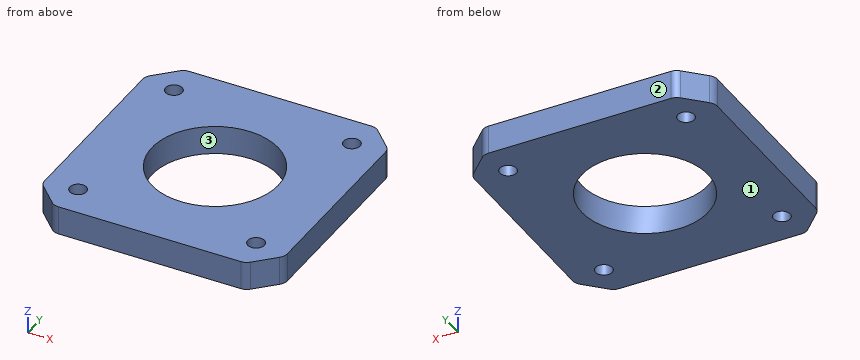
from build123d import *

# Parameters (mm, degrees)
SKETCH1_R           = 1.45
SKETCH1_R_2         = 11
BOSS_EXTRUDE1_DEPTH = 5


with BuildPart() as part:
    # Sketch1 → Boss-Extrude1 (new body)
    with BuildSketch(Plane.XY):
        with BuildLine():
            Line((-20.564213562, -17.28137085), (-17.28137085, -20.564213562))
            ThreePointArc((-17.28137085, -20.564213562), (-16.632524152, -20.997759065), (-15.867157288, -21.15))
            Line((-15.867157288, -21.15), (15.867157288, -21.15))
            ThreePointArc((15.867157288, -21.15), (16.632524152, -20.997759065), (17.28137085, -20.564213562))
            Line((17.28137085, -20.564213562), (20.564213562, -17.28137085))
            ThreePointArc((20.564213562, -17.28137085), (20.997759065, -16.632524152), (21.15, -15.867157288))
            Line((21.15, -15.867157288), (21.15, 15.867157288))
            ThreePointArc((21.15, 15.867157288), (20.997759065, 16.632524152), (20.564213562, 17.28137085))
            Line((20.564213562, 17.28137085), (17.28137085, 20.564213562))
            ThreePointArc((17.28137085, 20.564213562), (16.632524152, 20.997759065), (15.867157288, 21.15))
            Line((15.867157288, 21.15), (-15.867157288, 21.15))
            ThreePointArc((-15.867157288, 21.15), (-16.632524152, 20.997759065), (-17.28137085, 20.564213562))
            Line((-17.28137085, 20.564213562), (-20.564213562, 17.28137085))
            ThreePointArc((-20.564213562, 17.28137085), (-20.997759065, 16.632524152), (-21.15, 15.867157288))
            Line((-21.15, 15.867157288), (-21.15, -15.867157288))
            ThreePointArc((-21.15, -15.867157288), (-20.997759065, -16.632524152), (-20.564213562, -17.28137085))
        make_face()
        with Locations((-15.5, 15.5)):
            Circle(SKETCH1_R, mode=Mode.SUBTRACT)
        with Locations((15.5, 15.5)):
            Circle(SKETCH1_R, mode=Mode.SUBTRACT)
        with Locations((15.5, -15.5)):
            Circle(SKETCH1_R, mode=Mode.SUBTRACT)
        with Locations((-15.5, -15.5)):
            Circle(SKETCH1_R, mode=Mode.SUBTRACT)
        Circle(SKETCH1_R_2, mode=Mode.SUBTRACT)
    extrude(amount=BOSS_EXTRUDE1_DEPTH)


solid = part.part
Design review of the part built by this model. Coordinates are the model's own, in mm. Face numbers are marked on the shaded views. Give positions to 0.01 mm unless a question says otherwise; leave off trailing zeros. Write each loop counter-clockwise with the first axis right and the second up, starting at its lowest first coordinate (ties: lowest second). Pieces come first, ordered by that corner, then holes. Notation, with made-up numbers: M 87,29 L 129,29 A19 ccw 129,33 Z; hole C 21,36 d2. An arc over 180 degrees is marked long. Answer as a JSON object with one key per item and string values. Group by question number.
1) We need section A-A (y = 0). Give the boundary of the cut face in (x, z).
2) Mouldability with a two-part tool opening along Y and no side actions: class the marked faces 1, 2 and 3 as released by +Y, released by -Y, zero draft, split by the parting line, or undercut.
3) Clearance check with flat-ended pins moving along their axes: pin 1 Ø1 at (x, z) = (16, 4.5) entering from -Y; pin 2 Ø2.5 at (x, y) = (-15.5, -15.5) entering from -Z. State where each tip first meets the part, or that it passes through.
4) For line 1 along Y through (x, z) = (-15.5, 2.95); line 2 along Y through (x, z) = (0, 2); line 3 along Y through (x, z) = (-2.5, 2.6), list the stretches that pass through material, from the lowest coordinate up.
5) We need section C-C (z = 2.25). Give the boundary of the cut face in (x, y), and give its area (3 significant figures).
Answer key:
{
 "1": {"outline": "M -21.15,0 L -11,0 L -11,5 L -21.15,5 Z; M 11,0 L 21.15,0 L 21.15,5 L 11,5 Z"},
 "2": {"face 1": "zero draft", "face 2": "released by +Y", "face 3": "undercut"},
 "3": {"pin 1": "stops at y = -21.15", "pin 2": "passes through"},
 "4": {"line 1": "y = -21.15 to -16.95, -14.05 to 14.05, 16.95 to 21.15", "line 2": "y = -21.15 to -11, 11 to 21.15", "line 3": "y = -21.15 to -10.71, 10.71 to 21.15"},
 "5": {"outline": "M -21.15,-15.87 A2 ccw -20.56,-17.28 L -17.28,-20.56 A2 ccw -15.87,-21.15 L 15.87,-21.15 A2 ccw 17.28,-20.56 L 20.56,-17.28 A2 ccw 21.15,-15.87 L 21.15,15.87 A2 ccw 20.56,17.28 L 17.28,20.56 A2 ccw 15.87,21.15 L -15.87,21.15 A2 ccw -17.28,20.56 L -20.56,17.28 A2 ccw -21.15,15.87 Z; hole C -15.5,-15.5 d2.9; hole C -15.5,15.5 d2.9; hole C 0,0 d22; hole C 15.5,-15.5 d2.9; hole C 15.5,15.5 d2.9", "area": "1,340 mm²"}
}
